The listing builds one solid part. Answer for the finished solid, in the listing's coordinates (mm). A direction names the side the tool comes from. Coordinates: 2 decimals unless noted, no trailing zeros. Write each loop counter-clockwise with the first axis right and the second up, starting at its lowest first coordinate (ties: lowest second). Pieces come first, ordered by that corner, then holes.
from build123d import *

# Parameters (mm, degrees)
SKETCH1_R           = 85.725
BOSS_EXTRUDE1_DEPTH = 114.3
CUT_EXTRUDE1_DEPTH  = 152.4
SKETCH3_R           = 2.778125
CUT_EXTRUDE2_DEPTH  = 12.7
SKETCH4_R           = 6.985
CUT_EXTRUDE3_DEPTH  = 6.096


with BuildPart() as part:
    # Sketch1 → Boss-Extrude1 (new body)
    with BuildSketch(Plane(origin=(0, 0, 0), x_dir=(1, 0, 0), z_dir=(0, 1, 0))):
        Circle(SKETCH1_R)
    extrude(amount=BOSS_EXTRUDE1_DEPTH)

    # Sketch2 → Cut-Extrude1 (cut)
    with BuildSketch(Plane(origin=(0, 114.3, 0), x_dir=(1, 0, 0), z_dir=(0, 1, 0))):
        Polygon((85.724933621, -0.10668), (0, -85.725), (-45.627504124, -96.719379999), (-137.428949547, 46.173941299), (19.12530113, 101.910533163), (109.833872203, 30.600481808), align=None)
    extrude(amount=-CUT_EXTRUDE1_DEPTH, mode=Mode.SUBTRACT)

    # Sketch3 → Cut-Extrude2 (cut)
    with BuildSketch(Plane(origin=(42.862466811, 0, 42.91584), x_dir=(-0.707546622, 0, 0.706666667), z_dir=(-0.706666667, 0, -0.707546622))):
        with Locations((-37.719, 87.122)):
            Circle(SKETCH3_R)
        with Locations((-14.859, 87.122)):
            Circle(SKETCH3_R)
        with Locations((-37.719, 29.21)):
            Circle(SKETCH3_R)
        with Locations((-14.859, 29.21)):
            Circle(SKETCH3_R)
        with Locations((6.643736743, 73.636006083)):
            Circle(SKETCH3_R)
        with Locations((26.963736743, 73.636006083)):
            Circle(SKETCH3_R)
    extrude(amount=-CUT_EXTRUDE2_DEPTH, mode=Mode.SUBTRACT)

    # Sketch4 → Cut-Extrude3 (cut)
    with BuildSketch(Plane(origin=(0, 0, 0), x_dir=(-1, 0, 0), z_dir=(0, -1, 0))):
        with Locations((-51.720733405, -51.785137083)):
            Circle(SKETCH4_R)
    extrude(amount=-CUT_EXTRUDE3_DEPTH, mode=Mode.SUBTRACT)


solid = part.part
Q1. Determine the mould class of faces 4 (the face through (43, 0, 49)), 5 (the face through (62.38, 87.16, 41.37)), 6 (the face through (59.909, 56.35, 61.316)) for opening direction Z: released by +Z, released by -Z, zero draft, split by the parting line, or undercut.
Answers below:
face 4: zero draft
face 5: undercut
face 6: released by +Z
Q2. Given pin 1 (2 mm diameter, centred on x = 56.5, y = 12.5, fed in from +Z); pin 2 (5 mm diameter, centred on y = 25, z = 39, fed in from -X); pin 3 (1.5 mm diameter, centred on x = 66.5, y = 21.5, fed in from -Z), each flat-ended and moving along its own axis, determine where each tip first touches the part or whether it passes through.
Answers below:
pin 1: stops at z = 65.33
pin 2: stops at x = 44.28
pin 3: stops at z = 18.56
Q3. Find the intervals of material crossed by probe 1 along Z at (x, y) = (58, 63); probe 2 along Y at (x, z) = (26, 65); probe 3 along Z at (x, y) = (72, 25.5), in increasing order.
Answers below:
probe 1: z = 27.8 to 63.13
probe 2: y = 0 to 70.92, 76.35 to 114.3
probe 3: z = 13.81 to 46.53
Q4. The part is cut by section B-B, the plane x = 73.5. State how many separate pieces and enclosed holes the cut face has, then the cut area to 3 significant figures.
Answers below:
separate pieces: 1
enclosed holes: 2
area: 3,570 mm2
Q5. The part is cut by section A-A, the plane y = 65. Write down the section's boundary in (x, z) (3 decimals).
Answers below:
outline: (0, 85.725) - (85.725, 0.107) arc R85.725 ccw to start
Q6. The part is cut by section C-C, the plane z = 79.5. Write down the section's boundary in (x, y).
Answers below:
outline: (6.23, 0) - (32.07, 0) - (32.07, 114.3) - (6.23, 114.3) - close
Q7. Which of the six approach directions +Z, -Z, +X, -X, +Y, -Y give full straight-line access (tool end or side, diameter ignored) to faces 1 (the face through (78.55, 87.16, 25.22)), 2 (the face through (43.46, 57.95, 42.32)), 3 (the face through (52, 6.096, 52))?
Answers below:
face 1: none
face 2: -Z, -X, +Y, -Y
face 3: -Y
